from build123d import *

# Parameters (mm, degrees)
SKETCH_1_R      = 1.5
EXTRUDE_1_DEPTH = 3
FILLET_1_R      = 5
FILLET_2_R      = 10
FILLET_6_R      = 5
FILLET_7_R      = 5


with BuildPart() as part:
    # 草图1 → 凸台-拉伸1 (new body)
    with BuildSketch(Plane(origin=(0, 0, 0), x_dir=(1, 0, 0), z_dir=(0, 1, 0))):
        with BuildLine():
            Line((-46.499999325, -0.004997817), (-46.499999325, -6.504997817))
            Line((-46.499999325, -6.504997817), (-27.499999325, -6.504997817))
            Line((-27.499999325, -6.504997817), (-27.499999325, -32.5))
            Line((-27.499999325, -32.5), (6.5, -32.5))
            Line((6.5, -32.5), (6.5, -24.140215409))
            ThreePointArc((6.5, -24.140215409), (18.98987541, 16.25990873), (-22.851559401, 10.139340853))
            ThreePointArc((-22.851559401, 10.139340853), (-38.019140611, 12.86120129), (-46.499999325, -0.004997817))
        make_face()
        with Locations(Location((-32.499999325, 5.995002183, 0), (0, 0, 270))):
            Circle(SKETCH_1_R, mode=Mode.SUBTRACT)
        with Locations(Location((-27.303846902, -3.004997817, 0), (0, 0, 270))):
            Circle(SKETCH_1_R, mode=Mode.SUBTRACT)
        with Locations(Location((-3.5, -28.5, 0), (0, 0, 270))):
            Circle(SKETCH_1_R, mode=Mode.SUBTRACT)
        with Locations(Location((-37.696151748, -3.004997817, 0), (0, 0, 270))):
            Circle(SKETCH_1_R, mode=Mode.SUBTRACT)
        with Locations(Location((-21.058777701, -21.409353158, 0), (0, 0, 270))):
            Circle(SKETCH_1_R, mode=Mode.SUBTRACT)
        with Locations(Location((0, 15.5, 0), (0, 0, 270))):
            Circle(SKETCH_1_R, mode=Mode.SUBTRACT)
        with Locations(Location((13.423393759, 7.75, 0), (0, 0, 270))):
            Circle(SKETCH_1_R, mode=Mode.SUBTRACT)
        with Locations(Location((13.423393759, -7.75, 0), (0, 0, 270))):
            Circle(SKETCH_1_R, mode=Mode.SUBTRACT)
        with Locations(Location((0, -15.5, 0), (0, 0, 270))):
            Circle(SKETCH_1_R, mode=Mode.SUBTRACT)
        with Locations(Location((-13.423393759, -7.75, 0), (0, 0, 270))):
            Circle(SKETCH_1_R, mode=Mode.SUBTRACT)
        with Locations(Location((-13.423393759, 7.75, 0), (0, 0, 270))):
            Circle(SKETCH_1_R, mode=Mode.SUBTRACT)
        with BuildLine():
            ThreePointArc((-12.313744557, 4.167936537), (-13, 0), (-12.313744557, -4.167936537))
            ThreePointArc((-12.313744557, -4.167936537), (-10.175798494, -5.875), (-9.766411201, -8.580047334))
            ThreePointArc((-9.766411201, -8.580047334), (-6.5, -11.258330249), (-2.547333356, -12.747983871))
            ThreePointArc((-2.547333356, -12.747983871), (0, -11.75), (2.547333356, -12.747983871))
            ThreePointArc((2.547333356, -12.747983871), (6.5, -11.258330249), (9.766411201, -8.580047334))
            ThreePointArc((9.766411201, -8.580047334), (10.175798494, -5.875), (12.313744557, -4.167936537))
            ThreePointArc((12.313744557, -4.167936537), (13, 0), (12.313744557, 4.167936537))
            ThreePointArc((12.313744557, 4.167936537), (10.175798494, 5.875), (9.766411201, 8.580047334))
            ThreePointArc((9.766411201, 8.580047334), (6.5, 11.258330249), (2.547333356, 12.747983871))
            ThreePointArc((2.547333356, 12.747983871), (0, 11.75), (-2.547333356, 12.747983871))
            ThreePointArc((-2.547333356, 12.747983871), (-6.5, 11.258330249), (-9.766411201, 8.580047334))
            ThreePointArc((-9.766411201, 8.580047334), (-10.175798494, 5.875), (-12.313744557, 4.167936537))
        make_face(mode=Mode.SUBTRACT)
    extrude(amount=EXTRUDE_1_DEPTH)

    # 圆角1
    fillet_1_edges = [part.edges().sort_by_distance(p)[0] for p in [
        (-27.499999325, 1.5, 32.5),
        (-27.499999325, 1.5, 6.504997817),
        (-46.499999325, 1.5, 6.504997817),
    ]]
    fillet(fillet_1_edges, radius=FILLET_1_R)

    # 圆角2
    fillet_2_edges = [part.edges().sort_by_distance(p)[0] for p in [
        (-22.851559401, 1.5, -10.139340853),
    ]]
    fillet(fillet_2_edges, radius=FILLET_2_R)

    # 圆角6
    fillet_6_edges = [part.edges().sort_by_distance(p)[0] for p in [
        (6.5, 1.5, 24.140215409),
    ]]
    fillet(fillet_6_edges, radius=FILLET_6_R)

    # 圆角7
    fillet_7_edges = [part.edges().sort_by_distance(p)[0] for p in [
        (6.5, 1.5, 32.5),
    ]]
    fillet(fillet_7_edges, radius=FILLET_7_R)


solid = part.part
Part model, mm, in its own coordinate system. A direction names the side the tool comes from. Round coordinates to 2 decimals unless told otherwise and drop trailing zeros. Loops run counter-clockwise (first coordinate to the right, second up) from the corner with the lowest first, then second, coordinate; pieces in that order, holes last. Notation, with made-up numbers: (-35, -25.5) - (-26, -25.5) arc R27 cw to (-26, 7.5) - close; hole circle Ø8 at (83, 7.25). An arc over 180 degrees is marked (long way). Answer as a JSON object with one key per item and string values.
Item 1: Band-saw the part on A-A on z = 15.5. List the corners of the cut face in (x, y), plus the area to 3 significant figures.
Output:
{"outline": "(-27.5, 0) - (-1.5, 0) - (-1.5, 3) - (-27.5, 3) - close; (1.5, 0) - (19.62, 0) - (19.62, 3) - (1.5, 3) - close", "area": "132 mm2"}
Item 2: Band-saw the part on D-D on y = 0.7. State how many separate pieces and enclosed holes the cut face has, plus the area to 3 significant figures.
Output:
{"separate pieces": "1", "enclosed holes": "12", "area": "2,220 mm2"}
Item 3: Pin check, flat tips, straight feed: pin 1 (2.5 mm diameter, centred on x = -13.42, z = -7.75, fed in from -Y); pin 2 (1.5 mm diameter, centred on x = 7, y = 2, fed in from -Z). Stop position of each tip, or through.
Output:
{"pin 1": "through", "pin 2": "z = -24.21"}
Item 4: Band-saw the part on C-C on z = 3. List the corners of the cut face in (x, y).
Output:
{"outline": "(-46.27, 0) - (-39.2, 0) - (-39.2, 3) - (-46.27, 3) - close; (-36.2, 0) - (-28.8, 0) - (-28.8, 3) - (-36.2, 3) - close; (-25.8, 0) - (-12.65, 0) - (-12.65, 3) - (-25.8, 3) - close; (12.65, 0) - (24.82, 0) - (24.82, 3) - (12.65, 3) - close"}
Item 5: Pull direction X, two halves, no side cores. Call faces 1 (the face through (-6.448, 1.479, -11.288)), 2 (the face through (-37, 1, 6.505)), 3 (the face through (6.448, 1.479, 11.288)), 4 (the face through (-26.07, 1.52, 31)): pulls with the +X half, pulls with the -X half, needs draft (parallel to the pull), parting line crosses it, or undercut.
Output:
{"face 1": "undercut", "face 2": "needs draft", "face 3": "undercut", "face 4": "pulls with the -X half"}
Item 6: Wall check: L1, parallel to X at y = 1.9, z = 7.75; L2, parallel to X at y = 1.55, z = -7.75; L3, parallel to Z at x = 14, y = 1.15. Give the ranges that are in metal, low to high.
Output:
{"L1": "-29.2 to -14.92, -11.92 to -9.67, 9.67 to 11.92, 14.92 to 23.77", "L2": "-44.16 to -14.92, -11.92 to -9.67, 9.67 to 11.92, 14.92 to 23.77", "L3": "-20.71 to -9.13, -6.37 to 6.37, 9.13 to 20.71"}
Item 7: Band-saw the part on B-B on x = -3.5. List the corners of the cut face in (y, z), plus the area to 3 significant figures.
Output:
{"outline": "(0, -24.75) - (3, -24.75) - (3, -12.52) - (0, -12.52) - close; (0, 12.52) - (3, 12.52) - (3, 27) - (0, 27) - close; (0, 30) - (3, 30) - (3, 32.5) - (0, 32.5) - close", "area": "87.6 mm2"}
Item 8: Tool access for faces 5 (the face through (10.156, 1.479, 5.909)), 6 (the face through (-11, 1, 32.5)): list every direction of +Z, -Z, +X, -X, +Y, -Y with a clear straight run to the whole face (end or side of a thin tool).
Output:
{"face 5": "+Y, -Y", "face 6": "+Z, +X, -X, +Y, -Y"}
